from build123d import *

# Parameters (mm, degrees)
F1_DEPTH = 3


with BuildPart() as f1:
    # F0 (on Top) → F1 (new body)
    with BuildSketch(Plane.XY):
        Polygon((0.17165, -143.402397), (11.122826, -19.212155), (124.275944, -71.552546), (22.199627, 0.026572), (124.104294, 71.849852), (11.076801, 19.238727), (-0.17165, 143.402397), (-11.122826, 19.212155), (-124.275944, 71.552546), (-22.199627, -0.026572), (-124.104294, -71.849852), (-11.076801, -19.238727), align=None)
        Polygon((-10.397267, -0.012445), (-58.205037, 33.511865), (-5.209411, 8.998074), (-0.080393, 67.162973), (5.187855, 9.01052), (58.124645, 33.651109), (10.397267, 0.012445), (58.205037, -33.511865), (5.209411, -8.998074), (0.080393, -67.162973), (-5.187855, -9.01052), (-58.124645, -33.651109), align=None, mode=Mode.SUBTRACT)
    extrude(amount=F1_DEPTH)


solid = f1.part
Model file for the job. Use its own axes, mm. A direction names the side the tool comes from. Give positions to 0.01 mm unless a question says otherwise; leave off trailing zeros. Order: outer loops, then holes, each group sorted by start corner. A loop starts at its lowest first (then second) coordinate and runs counter-clockwise, first axis right, second up. Notation, with made-up numbers: (41.25, 67.25) - (48.25, 67.25) arc R17 ccw to (48.25, 89.25) - close; hole circle Ø11 at (48.5, -32). An arc over 180 degrees is marked (long way). Write item = value, one per line. Start each with the question number.
1. Cut at D-D, the plane x = -36. List the corners of the cut face in (y, z).
2. Drop flat-ended pins along their axis: P1, Ø1, axis at x = -23, z = 1.5, coming from the +Y side; P2, Ø1.5, axis at x = 74.5, z = 1, coming from the +Y side; P3, Ø1, axis at y = 99.5, z = 2, coming from the -X side. Give the stop position or say it passes through.
3. Two-plate mould, pull along Y, no slides. Class faces 4 (the flat face through (-31.29, -21.16, 1.48)), 5 (the flat face through (-66.907, 45.016, 1.479)), 6 (the flat face through (5.57, -82.18, 1.48)), 7 (the flat face through (-32.078, 21.427, 1.479)): pulls with the +Y half, pulls with the -Y half, needs draft (parallel to the pull), parting line crosses it, or undercut.
4. Cut at A-A, the plane z = 0.7. List the corners of the cut face in (x, y), and give its area (3 significant figures).
5. Cut at C-C, the plane y = 49. List the corners of the cut face in (x, z).
6. Probe line 1 along Y through (x, z) = (-46, 2.85); line 2 along Y through (x, z) = (-35.5, 1.7); line 3 along X through (y, z) = (26.5, 2.6). List the from-to ranges inside material, lowest first.
7. Cut at B-B, the plane x = 85.5. List the corners of the cut face in (y, z), and give its area (3 significant figures).
8. Which spindle directions (+Z, -Z, +X, -X, +Y, -Y) get a long thin tool onto all of the face, cutting with end or side? Do faces 1 (the flat face through (72.439, 35.435, 1.479)), 2 (the flat face through (-68.38, -45.91, 1.48)), 3 (the flat face through (-73.95, 36.26, 1.48)). Say none if no direction does.
Taken from the geometry:
q1.outline = (-30.84, 0) - (-23.35, 0) - (-23.35, 3) - (-30.84, 3) - close; (-18.06, 0) - (-9.75, 0) - (-9.75, 3) - (-18.06, 3) - close; (9.65, 0) - (17.94, 0) - (17.94, 3) - (9.65, 3) - close; (23.24, 0) - (30.72, 0) - (30.72, 3) - (23.24, 3) - close
q2.P1 = 24.94
q2.P2 = 49.11
q2.P3 = -4.09
q3.face_4 = undercut
q3.face_5 = pulls with the +Y half
q3.face_6 = pulls with the -Y half
q3.face_7 = undercut
q4.outline = (-124.28, 71.55) - (-22.2, -0.03) - (-124.1, -71.85) - (-11.08, -19.24) - (0.17, -143.4) - (11.12, -19.21) - (124.28, -71.55) - (22.2, 0.03) - (124.1, 71.85) - (11.08, 19.24) - (-0.17, 143.4) - (-11.12, 19.21) - close; hole (-58.21, 33.51) - (-10.4, -0.01) - (-58.12, -33.65) - (-5.19, -9.01) - (0.08, -67.16) - (5.21, -9) - (58.21, -33.51) - (10.4, 0.01) - (58.12, 33.65) - (5.19, 9.01) - (-0.08, 67.16) - (-5.21, 9) - close
q4.area = 7,460 mm²
q5.outline = (-92.11, 0) - (-75.52, 0) - (-75.52, 3) - (-92.11, 3) - close; (-8.5, 0) - (-1.68, 0) - (-1.68, 3) - (-8.5, 3) - close; (1.57, 0) - (8.38, 0) - (8.38, 3) - (1.57, 3) - close; (75.01, 0) - (91.68, 0) - (91.68, 3) - (75.01, 3) - close
q6.line_1 = -35.49 to -28.01, -25.11 to -16.8, 16.66 to 24.95, 27.87 to 35.35
q6.line_2 = -30.61 to -23.12, -17.71 to -9.4, 9.3 to 17.59, 23.01 to 30.49
q6.line_3 = -60.03 to -48.21, -43.05 to -26.88, -10.48 to -3.67, 3.6 to 10.42, 26.68 to 42.76, 47.98 to 59.76
q7.outline = (-53.62, 0) - (-44.36, 0) - (-44.36, 3) - (-53.62, 3) - close; (44.64, 0) - (53.88, 0) - (53.88, 3) - (44.64, 3) - close
q7.area = 55.5 mm²
q8.face_1 = +Z, -Z, +X
q8.face_2 = +Z, -Z, -Y
q8.face_3 = +Z, -Z, -X
